Can you work these out from the model? Positions are in its coordinate system, mm. A direction names the side the tool comes from. Round coordinates to 2 decimals unless told otherwise and drop trailing zeros. Write each loop counter-clockwise with the first axis right and the second up, starting at its lowest first coordinate (ties: lowest second). Pieces come first, ordered by that corner, then holes. Notation, with made-up numbers: M 58.5,4 L 107.5,4 A25 cw 107.5,17 Z; hole C -9.5,8 d6. An arc over 180 degrees is marked long. Answer in a Markdown table with one row per item. Add a question column.
(1) If I drill on probe 1 along X at (y, z) = (1.4, 0) (3 decimals); probe 2 along Z at (x, y) = (-8.5, 2.3); probe 3 along X at (y, z) = (0.2, -6), over which ranges is the centre line in solid material (lowest first)?
(2) Suppose I cut it at B-B, the plane x = 0. Write out the boundary of the cut face in (y, z) (3 decimals), then the cut area to 4 significant figures.
(3) Suppose I cut it at A-A, the plane z = 0. Write out the boundary of the cut face in (x, y) (3 decimals), then the cut area to 4 significant figures.
(4) Suppose I cut it at D-D, the plane x = 9. Write out the boundary of the cut face in (y, z), then the cut area to 3 significant figures.
(5) Suppose I cut it at C-C, the plane y = 2.35. Write out the boundary of the cut face in (x, z) (3 decimals).
(6) If we mould it in two halves opening along Z, with no side actions, what happens to faces 3 (the face through (10.5, 1, 0)), 4 (the face through (0.74, 1.48, 2.36)), 5 (the face through (-12.6, 1.5, -12.8)), 6 (the face through (0, 1, 17.9))? For each: released by +Z, released by -Z, zero draft, split by the parting line, or undercut.
(7) For faces 1 (the face through (-12, 1, 1.425)), 2 (the face through (-12.8, 1.5, 12.6)), which set-ups out of +Z, -Z, +X, -X, +Y, -Y let a thin tool reach every point of the face, with its end or its side?
(8) I'm going to push flat-ended pins straight in: pin 1 (1.5 mm diameter, centred on y = 2, z = -12, fed in from +X); pin 2 (1.5 mm diameter, centred on x = -12, y = 1.5, fed in from +Z); pin 3 (1 mm diameter, centred on y = 1.5, z = -4.5, fed in from +X). Where does each tip first touch, or does it pass through?
from build123d import *

# Parameters (mm, degrees)
SKETCH1_R           = 2.475
SKETCH1_W           = 2.85
SKETCH1_H           = 3.5
SKETCH1_W_2         = 3.5
SKETCH1_H_2         = 2.85
BOSS_EXTRUDE1_DEPTH = 3


with BuildPart() as part:
    # Sketch1 → Boss-Extrude1 (new body)
    with BuildSketch(Plane(origin=(0, 0, 0), x_dir=(1, 0, 0), z_dir=(0, 1, 0))):
        with BuildLine():
            Line((-1.5, -17.9), (1.5, -17.9))
            ThreePointArc((1.5, -17.9), (12.701574706, -12.701574706), (17.9, -1.5))
            Line((17.9, -1.5), (17.9, 1.5))
            ThreePointArc((17.9, 1.5), (12.701574706, 12.701574706), (1.5, 17.9))
            Line((1.5, 17.9), (-1.5, 17.9))
            ThreePointArc((-1.5, 17.9), (-12.701574706, 12.701574706), (-17.9, 1.5))
            Line((-17.9, 1.5), (-17.9, -1.5))
            ThreePointArc((-17.9, -1.5), (-12.701574706, -12.701574706), (-1.5, -17.9))
        make_face()
        with Locations(Location((0, 0, 0), (0, 0, 270))):
            Circle(SKETCH1_R, mode=Mode.SUBTRACT)
        with Locations((0, -12.25)):
            Rectangle(SKETCH1_W, SKETCH1_H, mode=Mode.SUBTRACT)
        with Locations((-12.25, 0)):
            Rectangle(SKETCH1_W_2, SKETCH1_H_2, mode=Mode.SUBTRACT)
        with Locations((0, 12.25)):
            Rectangle(SKETCH1_W, SKETCH1_H, mode=Mode.SUBTRACT)
        with Locations((12.25, 0)):
            Rectangle(SKETCH1_W_2, SKETCH1_H_2, mode=Mode.SUBTRACT)
    extrude(amount=BOSS_EXTRUDE1_DEPTH)


solid = part.part
Calculated:
| question | item | result |
|---|---|---|
| 1 | probe 1 | -17.9 to -14, -10.5 to -2.475, 2.475 to 10.5, 14 to 17.9 |
| 1 | probe 2 | -15.82 to 15.82 |
| 1 | probe 3 | -16.93 to 16.93 |
| 2 | outline | M 0,-17.9 L 3,-17.9 L 3,-14 L 0,-14 Z; M 0,-10.5 L 3,-10.5 L 3,-2.475 L 0,-2.475 Z; M 0,2.475 L 3,2.475 L 3,10.5 L 0,10.5 Z; M 0,14 L 3,14 L 3,17.9 L 0,17.9 Z |
| 2 | area | 71.55 mm² |
| 3 | outline | M -17.9,0 L -14,0 L -14,3 L -17.9,3 Z; M -10.5,0 L -2.475,0 L -2.475,3 L -10.5,3 Z; M 2.475,0 L 10.5,0 L 10.5,3 L 2.475,3 Z; M 14,0 L 17.9,0 L 17.9,3 L 14,3 Z |
| 3 | area | 71.55 mm² |
| 4 | outline | M 0,-15.55 L 3,-15.55 L 3,15.55 L 0,15.55 Z |
| 4 | area | 93.3 mm² |
| 5 | outline | M -17.9,-1.5 A17.963 ccw -1.5,-17.9 L 1.5,-17.9 A17.963 ccw 17.9,-1.5 L 17.9,1.5 A17.963 ccw 1.5,17.9 L -1.5,17.9 A17.963 ccw -17.9,1.5 Z; hole M -14,-1.425 L -10.5,-1.425 L -10.5,1.425 L -14,1.425 Z; hole C 0,0 d4.95; hole M -1.425,-14 L 1.425,-14 L 1.425,-10.5 L -1.425,-10.5 Z; hole M -1.425,10.5 L 1.425,10.5 L 1.425,14 L -1.425,14 Z; hole M 10.5,-1.425 L 14,-1.425 L 14,1.425 L 10.5,1.425 Z |
| 6 | face 3 | undercut |
| 6 | face 4 | undercut |
| 6 | face 5 | released by -Z |
| 6 | face 6 | released by +Z |
| 7 | face 1 | +Y, -Y |
| 7 | face 2 | +Z, -X, +Y, -Y |
| 8 | pin 1 | x = 14 |
| 8 | pin 2 | z = 14 |
| 8 | pin 3 | x = 17.51 |
